For this review, use the dimensioned drawing (mm, ordinates from the lowest corner) and the shaded views. A direction names the side the tool comes from. Give positions to 0.01 mm unless a question says otherwise; leave off trailing zeros. Order: outer loops, then holes, each group sorted by start corner. A loop starts at its lowest first (then second) coordinate and runs counter-clockwise, first axis right, second up. Notation, with made-up numbers: (76.5, 47.5) - (84.5, 47.5) arc R27 ccw to (84.5, 67.5) - close; hole circle Ø11 at (54, 1). An arc over 180 degrees is marked (long way). One line per item, written item: value.
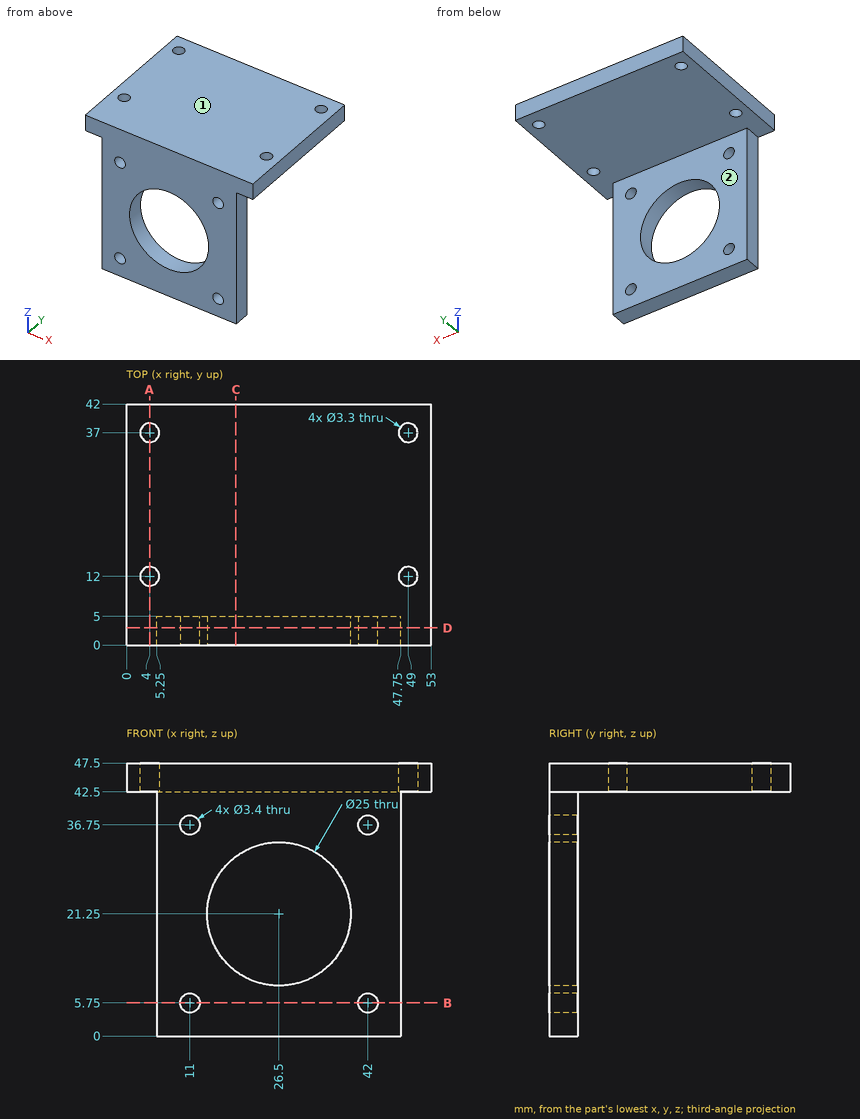
(1) Take a section at B-B (z = 5.75). Write out the cut boundary in (x, y).
Answers below:
outline: (5.25, 0) - (9.3, 0) - (9.3, 5) - (5.25, 5) - close; (12.7, 0) - (40.3, 0) - (40.3, 5) - (12.7, 5) - close; (43.7, 0) - (47.75, 0) - (47.75, 5) - (43.7, 5) - close
(2) Wall thickness on line 1 (Y direction, x = 49, z = 46.55); line 2 (Z direction, x = 42, y = 1.65); line 3 (X direction, y = 1.4, z = 5.75): over which ranges is each line inside the solid? List them lowest first. Write a range as from..to.
Answers below:
line 1: y = 0..10.35, 13.65..35.35, 38.65..42
line 2: z = 0..4.05, 7.45..35.05, 38.45..47.5
line 3: x = 5.25..9.3, 12.7..40.3, 43.7..47.75
(3) Take a section at D-D (y = 3). Write out the cut boundary in (x, z).
Answers below:
outline: (0, 42.5) - (5.25, 42.5) - (5.25, 0) - (47.75, 0) - (47.75, 42.5) - (53, 42.5) - (53, 47.5) - (0, 47.5) - close; hole circle Ø3.4 at (11, 5.75); hole circle Ø3.4 at (11, 36.75); hole circle Ø25 at (26.5, 21.25); hole circle Ø3.4 at (42, 5.75); hole circle Ø3.4 at (42, 36.75)
(4) Take a section at C-C (x = 19). Write out the cut boundary in (y, z), then the cut area to 4 significant figures.
Answers below:
outline: (0, 0) - (5, 0) - (5, 11.25) - (0, 11.25) - close; (0, 31.25) - (5, 31.25) - (5, 42.5) - (42, 42.5) - (42, 47.5) - (0, 47.5) - close
area: 322.5 mm^2
(5) Take a section at A-A (x = 4). Write out the cut boundary in (y, z).
Answers below:
outline: (0, 42.5) - (10.35, 42.5) - (10.35, 47.5) - (0, 47.5) - close; (13.65, 42.5) - (35.35, 42.5) - (35.35, 47.5) - (13.65, 47.5) - close; (38.65, 42.5) - (42, 42.5) - (42, 47.5) - (38.65, 47.5) - close
(6) For P1, Ø4, axis at x = 49, y = 12, coming from the -Z side; P2, Ø3, axis at x = 11, z = 5.75, coming from the -Y side; P3, Ø10, axis at y = 9.5, z = 16, coming from the -X side; P4, Ø4.5, axis at x = 42, z = 5.75, coming from the +Y side, all flat-tipped, find the tip position at first contact; note any pin that passes through.
Answers below:
P1: stops at z = 42.5
P2: passes through
P3: stops at x = 5.25
P4: stops at y = 5
(7) Machinability: for the marked faces 1 and 2, which of the approach directions +Z, -Z, +X, -X, +Y, -Y give a long, thin tool a straight path to every point of the face, cutting with its end or side? Answer none if there is none.
Answers below:
face 1: +Z, +X, -X, +Y, -Y
face 2: -Z, +X, -X, +Y
